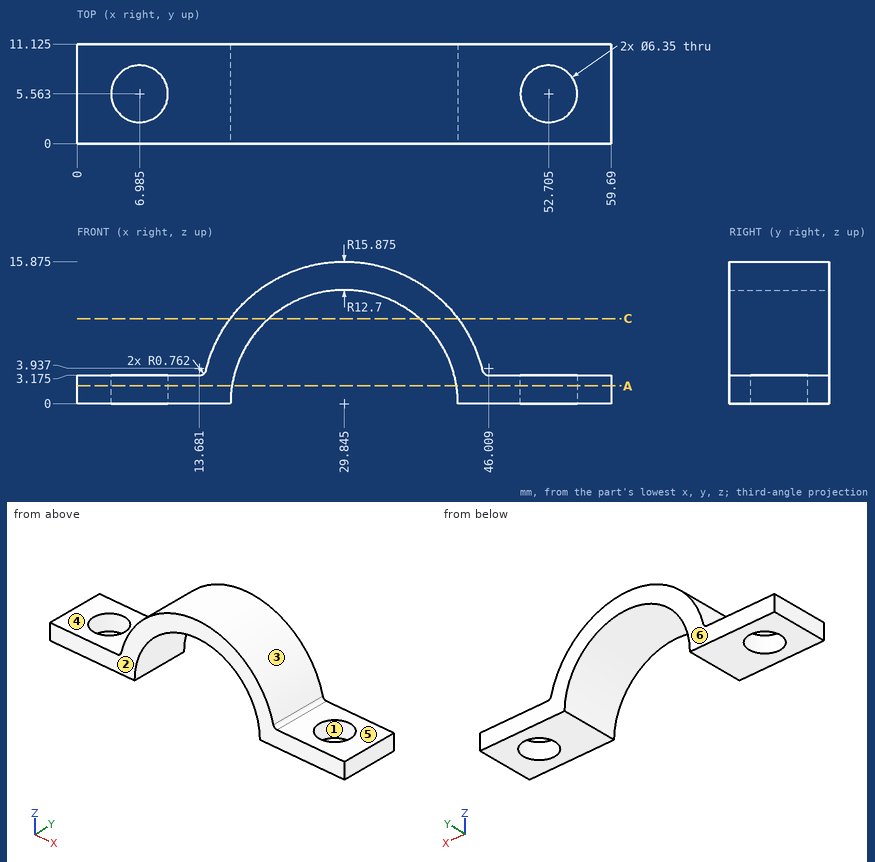
Geometry: see drawing. Coordinates: mm, zero at the bounding-box minimum. A direction names the side the tool comes from. Give positions to 0.01 mm unless a question says otherwise; leave off trailing zeros. Order: outer loops, then holes, each group sorted by start corner. A loop starts at its lowest first (then second) coordinate and runs counter-clockwise, first axis right, second up. Notation, with made-up numbers: M -34,39 L -12,39 A18 ccw -12,65 Z; hole C -26.75,33 d1. An arc over 180 degrees is marked long. Answer as a JSON object with one key per item and string values.
1. First-contact query: P1, Ø5, axis at x = 52.7, y = 5.56, coming from the -Z side; P2, Ø5, axis at x = 46, y = 5.5, coming from the +Z side (1 decimal); P3, Ø2, axis at y = 6, z = 4.5, coming from the -X side (1 decimal). Flat tips, straight axial feed; report the tip coordinate or a pass-through.
Result sheet:
{"P1": "through", "P2": "z = 8.1", "P3": "x = 14.3"}
2. Cut plane A-A, the plane z = 2. State how many separate pieces and enclosed holes the cut face has, and give its area (3 significant figures).
Result sheet:
{"separate pieces": "2", "enclosed holes": "2", "area": "322 mm²"}
3. Pull-direction query (X, two-part tool) for the marked faces 1, 2 and 3; classes: +X half, -X half, draft (parallel to the pull), parting line (faces both ways), or undercut.
Result sheet:
{"face 1": "undercut", "face 2": "draft", "face 3": "parting line"}
4. Cut plane C-C, the plane z = 9.5. Output: boundary loops of the cut face in (x, y) (1 decimal).
Result sheet:
{"outline": "M 17.1,0 L 21.4,0 L 21.4,11.1 L 17.1,11.1 Z; M 38.3,0 L 42.6,0 L 42.6,11.1 L 38.3,11.1 Z"}
5. Reachability of the marked faces 4, 5 and 6 from +Z, -Z, +X, -X, +Y, -Y: full face, straight path, thin tool, end or side. Return the list, or none.
Result sheet:
{"face 4": "+Z, -X, +Y, -Y", "face 5": "+Z, +X, +Y, -Y", "face 6": "+Z, -Z, +X, -X, +Y"}
6. Ray query, line 1 (X direction, y = 4.25, z = 3.75); line 2 (X direction, y = 1.5, z = 1) (1 decimal); line 3 (Z direction, x = 9, y = 2) (1 decimal). Return the intervals inside material, ascending. Write a range as [from, to].
Result sheet:
{"line 1": "[14.42, 17.71], [41.98, 45.27]", "line 2": "[0, 17.2], [42.5, 59.7]", "line 3": "[0, 3.2]"}
